Check sheet for the modelled part. Datum: model origin and axes. Units: mm. A direction names the side the tool comes from. Coordinates: 2 decimals unless noted, no trailing zeros. Write each loop counter-clockwise with the first axis right and the second up, starting at its lowest first coordinate (ties: lowest second). Pieces come first, ordered by that corner, then holes. Notation, with made-up numbers: (44, 31) - (63, 31) arc R32 cw to (63, 58) - close; hole circle Ø3 at (-36, 55.25). An arc over 180 degrees is marked (long way). Use one line per item in the form item = value. Start each with the question number.
1. Draft check along Y on faces 5 (the face through (57.153, -0.398, -55.366)), 6 (the face through (54.764, -0.398, -66.423)), 7 (the face through (61, 0, -72.339)). Enter one of: +Y half, -Y half, draft (parallel to the pull), parting line (faces both ways), or undercut.
2. Cross-section at A-A on z = -44.5. Record the boundary of the cut face in (x, y), then the cut area to 3 significant figures.
3. Cross-section at C-C on z = -70. Record the boundary of the cut face in (x, y) (3 decimals).
4. Tool access check on faces 1 (the face through (62.15, 0, -69)), 2 (the face through (62.15, 0, -59)), 3 (the face through (50.05, 0, -65)), 4 (the face through (55.05, 0, -45)). Record the directions out of +Z, -Z, +X, -X, +Y, -Y that give a thin tool (end or side, any length) a straight path to the whole face; none if there is none.
5. Go/stop test with flat-tipped pins: pin 1 Ø1.5 at (y, z) = (1, -67.5) entering from -X; pin 2 Ø1.6 at (y, z) = (1, -58.5) entering from +X; pin 3 Ø2.5 at (x, y) = (53.5, 0) entering from -Z. Record where each tip stops, or that it passes through.
6. Cross-section at B-B on x = 44. Record the boundary of the cut face in (y, z), then the cut area to 3 significant figures.
7. Scan lines: line 1 along Y through (x, z) = (53.5, -69) (3 decimals); line 2 along Z through (x, y) = (44, 0); line 3 along X through (y, z) = (0.6, -49). Record each from-to range of solid material in increasing order.
```python
from build123d import *

# Parameters (mm, degrees)
PAD004_DEPTH   = 5
SKETCH009_R    = 1.325
HOLE004_DEPTH  = 34.3965410847
SKETCH010_R    = 1.325
HOLE005_DEPTH  = 12
HOLE005_TIPS_R = 1.325


with BuildPart() as part:
    # Sketch008 → Pad004 (new body)
    with BuildSketch(Plane.XZ.offset(-2.5)):
        Polygon((49.95, -40.139016), (51.95, -40.139016), (51.95, -50.139016), (55.05, -50.139016), (55.05, -40.139016), (57.05, -40.139016), (57.05, -52.239016), (60.05, -55.239016), (72.15, -55.239016), (72.15, -57.239016), (62.15, -57.239016), (62.15, -60.339016), (72.15, -60.339016), (72.15, -62.339016), (66.3926406871, -62.339016), (62.15, -66.5816566871), (62.15, -72.339016), (60.15, -72.339016), (60.15, -62.339016), (57.05, -62.339016), (57.05, -72.339016), (50.05, -72.339016), (50.05, -57.239016), (39.95, -57.239016), (39.95, -55.239016), (49.95, -55.239016), (49.95, -52.139016), (39.95, -52.139016), (39.95, -50.139016), (45.7073593129, -50.139016), (49.95, -45.8963753129), align=None)
    extrude(amount=PAD004_DEPTH)

    # Sketch009 (on Face7 of Pad004) → Hole004 (cut, through all)
    with BuildSketch(Plane(origin=(64.3658283436, 0, -64.3658283436), x_dir=(0.7071067812, 0, 0.7071067812), z_dir=(0.7071067812, 0, -0.7071067812))):
        Circle(SKETCH009_R)
    extrude(amount=-HOLE004_DEPTH, mode=Mode.SUBTRACT)

    # Sketch010 (on Face17 of Hole004) → Hole005 (cut)
    with BuildSketch(Plane(origin=(0, 0, -72.339016), x_dir=(1, 0, 0), z_dir=(0, 0, -1))):
        with Locations((53.5, 0)):
            Circle(SKETCH010_R)
    extrude(amount=-HOLE005_DEPTH, mode=Mode.SUBTRACT)

    # Hole005 tips → Hole005 tip 1 section 0
    with BuildSketch(Plane(origin=(0, 0, -60.339016), x_dir=(1, 0, 0), z_dir=(0, 0, -1)), mode=Mode.PRIVATE) as hole005_tip_1_s0:
        with Locations((53.5, 0)):
            Circle(HOLE005_TIPS_R)
    loft([hole005_tip_1_s0.sketch, Vertex(53.5, 0, -59.5428756798)], mode=Mode.SUBTRACT)


solid = part.part
```
Final values:
q1.face_5 = undercut
q1.face_6 = undercut
q1.face_7 = draft
q2.outline = (49.95, -2.5) - (51.95, -2.5) - (51.95, 2.5) - (49.95, 2.5) - close; (55.05, -2.5) - (57.05, -2.5) - (57.05, 2.5) - (55.05, 2.5) - close
q2.area = 20.0 mm²
q3.outline = (50.05, -2.5) - (57.05, -2.5) - (57.05, 2.5) - (50.05, 2.5) - close; (60.15, -2.5) - (62.15, -2.5) - (62.15, 2.5) - (60.15, 2.5) - close; hole circle Ø2.65 at (53.5, 0)
q4.face_1 = -Z, +X, +Y, -Y
q4.face_2 = +X, +Y, -Y
q4.face_3 = -Z, -X, +Y, -Y
q4.face_4 = +Z, +Y, -Y
q5.pin_1 = 50.05
q5.pin_2 = 62.15
q5.pin_3 = -60.29
q6.outline = (-2.5, -57.24) - (2.5, -57.24) - (2.5, -55.24) - (-2.5, -55.24) - close; (-2.5, -52.14) - (2.5, -52.14) - (2.5, -50.14) - (-2.5, -50.14) - close
q6.area = 20.0 mm²
q7.line_1 = -2.5 to -1.325, 1.325 to 2.5
q7.line_2 = -57.24 to -55.24, -52.14 to -50.14
q7.line_3 = 46.85 to 47.33, 50.67 to 51.95, 55.05 to 57.05
